Source: CAD feature listing. Evaluate the final solid. Frame: model axes, mm. Coordinates: 2 decimals unless noted, no trailing zeros. Loops run counter-clockwise (first coordinate to the right, second up) from the corner with the lowest first, then second, coordinate; pieces in that order, holes last. Notation, with made-up numbers: (-14, 8.25) -> (19, 8.25) arc R11 cw to (19, 13.25) -> close; hole circle Ø7 at (27, 0.5). An arc over 180 degrees is marked (long way). Answer as CSV lines item,"result".
from build123d import *

# Parameters (mm, degrees)
SKETCH1_W           = 30
SKETCH1_H           = 7
BOSS_EXTRUDE1_DEPTH = 0.12
SKETCH2_W           = 0.5
SKETCH2_H           = 0.5
BOSS_EXTRUDE2_DEPTH = 0.1
SKETCH3_W           = 0.5
SKETCH3_H           = 0.5
BOSS_EXTRUDE3_DEPTH = 0.1


with BuildPart() as part:
    # Sketch1 → Boss-Extrude1 (new body)
    with BuildSketch(Plane(origin=(0, 0, 0), x_dir=(1, 0, 0), z_dir=(0, 1, 0))):
        with Locations((-15, -3.5)):
            Rectangle(SKETCH1_W, SKETCH1_H)
    extrude(amount=BOSS_EXTRUDE1_DEPTH)

    # Sketch2 → Boss-Extrude2 (add)
    with BuildSketch(Plane.XZ):
        with Locations((-0.25, 3.5)):
            Rectangle(SKETCH2_W, SKETCH2_H)
    extrude(amount=BOSS_EXTRUDE2_DEPTH)

    # Sketch3 → Boss-Extrude3 (add)
    with BuildSketch(Plane.XZ):
        with Locations((-29.75, 3.5)):
            Rectangle(SKETCH3_W, SKETCH3_H)
    extrude(amount=BOSS_EXTRUDE3_DEPTH)


solid = part.part
(1) Cut plane C-C (x = -5). Return the cut outline in (y, z), then the cut area to 3 significant figures.
Computed values:
outline,"(0, 0) -> (0.12, 0) -> (0.12, 7) -> (0, 7) -> close"
area,"0.840 mm^2"
(2) Cut plane D-D (z = 1.5). Return the cut outline in (x, y).
Computed values:
outline,"(-30, 0) -> (0, 0) -> (0, 0.12) -> (-30, 0.12) -> close"
(3) Cut plane A-A (y = -0.05). Return the cut outline in (x, z), then the cut area to 3 significant figures.
Computed values:
outline,"(-30, 3.25) -> (-29.5, 3.25) -> (-29.5, 3.75) -> (-30, 3.75) -> close; (-0.5, 3.25) -> (0, 3.25) -> (0, 3.75) -> (-0.5, 3.75) -> close"
area,"0.500 mm^2"
(4) Cut plane B-B (z = 3.5). Return the cut outline in (x, y), then the cut area to 3 significant figures.
Computed values:
outline,"(-30, -0.1) -> (-29.5, -0.1) -> (-29.5, 0) -> (-0.5, 0) -> (-0.5, -0.1) -> (0, -0.1) -> (0, 0.12) -> (-30, 0.12) -> close"
area,"3.70 mm^2"
(5) Pin query (flat end, axial travel): pin 1 Ø3 at (x, z) = (-22.5, 2.5) entering from -Y. Return the tip coordinate at first contact, or that it passes through.
Computed values:
pin 1,"y = 0"
